```python
from build123d import *

# Parameters (mm, degrees)
BOSS_EXTRUDE1_DEPTH = 3.175
SKETCH2_R           = 1.5
SKETCH2_R_2         = 1.500000048
CUT_EXTRUDE1_DEPTH  = 99.065877093
SKETCH4_R           = 1.5
CUT_EXTRUDE3_DEPTH  = 99.065877093
SKETCH5_W           = 82.55
SKETCH5_H           = 60.325
CUT_EXTRUDE4_DEPTH  = 99.065877093
SKETCH6_R           = 1.5
CUT_EXTRUDE5_DEPTH  = 99.065877093


with BuildPart() as part:
    # Sketch1 → Boss-Extrude1 (new body)
    with BuildSketch(Plane(origin=(0, 0, 0), x_dir=(1, 0, 0), z_dir=(0, 1, 0))):
        Polygon((-41.275, 0), (-36.368301991, -11.713851401), (-33.466950324, -10.424361771), (-17.857958519, -45.544593333), (-20.759310186, -46.834082962), (-15.601351667, -58.43948963), (-12.7, -60.325), (-5.08, -60.325), (-5.08, -57.15), (5.08, -57.15), (5.08, -60.325), (12.7, -60.325), (15.601351667, -58.43948963), (20.759310186, -46.834082962), (17.857958519, -45.544593333), (33.466950324, -10.424361771), (36.368301991, -11.713851401), (41.275, 0), (41.275, 25.4), (38.1, 25.4), (38.1, 50.8), (41.275, 50.8), (41.275, 88.9), (22.225, 88.9), (22.225, 85.725), (10.205057544, 85.725), (-10.205057544, 85.725), (-22.225, 85.725), (-22.225, 88.9), (-41.275, 88.9), (-41.275, 50.8), (-38.1, 50.8), (-38.1, 25.4), (-41.275, 25.4), align=None)
    extrude(amount=BOSS_EXTRUDE1_DEPTH)

    # Sketch2 → Cut-Extrude1 (cut, through all)
    with BuildSketch(Plane(origin=(0, 0, 0), x_dir=(-1, 0, 0), z_dir=(0, -1, 0))):
        with Locations(Location((39.6875, 76.2, 0), (0, 0, 90))):
            Circle(SKETCH2_R)
        with Locations(Location((-8.89, -58.7375, 0), (0, 0, 270))):
            Circle(SKETCH2_R_2)
        with Locations(Location((39.6875, 12.7, 0), (0, 0, 90))):
            Circle(SKETCH2_R_2)
        with Locations((37.496605417, -5.266403252)):
            Circle(SKETCH2_R_2)
        with Locations(Location((16.729655093, -51.992041481, 0), (0, 0, 90))):
            Circle(SKETCH2_R_2)
        with Locations(Location((8.89, -58.7375, 0), (0, 0, 90))):
            Circle(SKETCH2_R_2)
        with Locations(Location((-16.729655093, -51.992041481, 0), (0, 0, 270))):
            Circle(SKETCH2_R_2)
        with Locations((-37.496605417, -5.266403252)):
            Circle(SKETCH2_R_2)
        with Locations(Location((-39.6875, 12.7, 0), (0, 0, 270))):
            Circle(SKETCH2_R_2)
        with Locations(Location((-39.6875, 76.2, 0), (0, 0, 270))):
            Circle(SKETCH2_R)
    extrude(amount=-CUT_EXTRUDE1_DEPTH, mode=Mode.SUBTRACT)

    # Sketch4 → Cut-Extrude3 (cut, through all)
    with BuildSketch(Plane(origin=(0, 3.175, 0), x_dir=(1, 0, 0), z_dir=(0, 1, 0))):
        with Locations(Location((31.681488655, 11.305, 0), (0, 0, 270))):
            Circle(SKETCH4_R)
        with Locations(Location((31.681488655, 39.245, 0), (0, 0, 270))):
            Circle(SKETCH4_R)
        with Locations(Location((-20.388511345, 6.225, 0), (0, 0, 270))):
            Circle(SKETCH4_R)
        with Locations(Location((-19.118511345, 54.485, 0), (0, 0, 270))):
            Circle(SKETCH4_R)
    extrude(amount=-CUT_EXTRUDE3_DEPTH, mode=Mode.SUBTRACT)

    # Sketch5 → Cut-Extrude4 (cut, through all)
    with BuildSketch(Plane(origin=(0, 3.175, 0), x_dir=(1, 0, 0), z_dir=(0, 1, 0))):
        with Locations((0, -30.1625)):
            Rectangle(SKETCH5_W, SKETCH5_H)
    extrude(amount=-CUT_EXTRUDE4_DEPTH, mode=Mode.SUBTRACT)

    # Sketch6 → Cut-Extrude5 (cut, through all)
    with BuildSketch(Plane(origin=(0, 3.175, 0), x_dir=(1, 0, 0), z_dir=(0, 1, 0))):
        with Locations(Location((-30.099, 87.3125, 0), (0, 0, 270))):
            Circle(SKETCH6_R)
        with Locations(Location((30.099, 87.3125, 0), (0, 0, 270))):
            Circle(SKETCH6_R)
    extrude(amount=-CUT_EXTRUDE5_DEPTH, mode=Mode.SUBTRACT)


solid = part.part
```
Geometry check sheet. Reference: the model listing, model coordinates, mm. A direction names the side the tool comes from. Coordinates: 2 decimals unless noted, no trailing zeros. Order: outer loops, then holes, each group sorted by start corner. A loop starts at its lowest first (then second) coordinate and runs counter-clockwise, first axis right, second up.
Item 1: Mould release check, pull along Z, two halves, no side actions. Record for faces 1 (the flat face through (-1, 2, 0)), 2 (the flat face through (-22.225, 2, -87)), 3 (the cylindrical face through (-41.02, 1.57, -76.89)): released by +Z, released by -Z, zero draft, split by the parting line, or undercut.
Item 2: Scan lines: line 1 along X through (y, z) = (1.4, -11.5) (1 decimal); line 2 along Z through (x, y) = (-4.5, 2) (3 decimals); line 3 along Z through (x, y) = (-18.5, 1.3) (3 decimals). Record each from-to range of solid material in increasing order.
Item 3: Depth check by flat-ended pin: pin 1 (1.6 mm diameter, centred on y = 2, z = -42.5, fed in from -X). Enter the tip coordinate at first touch or a pass-through.
Item 4: Section check C-C (x = 1.5). Enter the section's corners in (y, z) (3 decimals), plus the area to 3 significant figures.
Item 5: Tool access check on faces 4 (the flat face through (-32, 2, -88.9)), 5 (the flat face through (22.225, 2, -87)), 6 (the flat face through (38.1, 2, -38)). Record the directions out of +Z, -Z, +X, -X, +Y, -Y that give a thin tool (end or side, any length) a straight path to the whole face; none if there is none.
Item 6: Section check A-A (z = -76.2). Count the separate pieces of the cut face and the enclosed holes in it, plus the area to 3 significant figures.
Check sheet entries:
1. face 1: released by +Z
1. face 2: zero draft
1. face 3: undercut
2. line 1: x = -41.3 to -40.6, -38.8 to 30.2, 33.2 to 38.8, 40.6 to 41.3
2. line 2: z = -85.725 to 0
2. line 3: z = -85.725 to -55.852, -53.118 to 0
3. pin 1: stops at x = -38.1
4. outline: (0, -85.725) - (3.175, -85.725) - (3.175, 0) - (0, 0) - close
4. area: 272 mm2
5. face 4: -Z, +X, -X, +Y, -Y
5. face 5: -Z, +Y, -Y
5. face 6: +X, +Y, -Y
6. separate pieces: 3
6. enclosed holes: 0
6. area: 243 mm2
